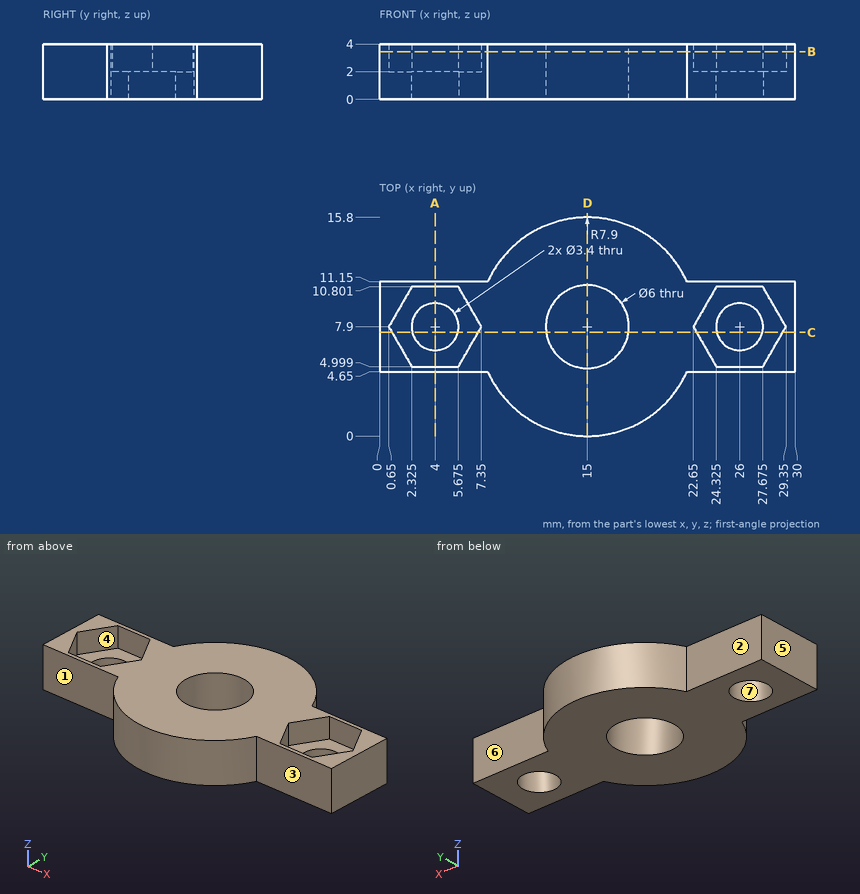
Drawing for the job (mm, zero at the part's lowest x, y, z). A direction names the side the tool comes from. Round coordinates to 2 decimals unless told otherwise and drop trailing zeros. Order: outer loops, then holes, each group sorted by start corner. A loop starts at its lowest first (then second) coordinate and runs counter-clockwise, first axis right, second up. Notation, with made-up numbers: (-28.75, 61) -> (23.25, 61) arc R19 ccw to (23.25, 69) -> close; hole circle Ø7 at (2.5, -24). An arc over 180 degrees is marked (long way). Write item = value, one per line. Start each with the question number.
(1) Cut at C-C, the plane y = 7.5. List the corners of the cut face in (x, z).
(2) Cut at A-A, the plane x = 4. List the corners of the cut face in (y, z).
(3) Cut at B-B, the plane z = 3.45. State how many separate pieces and enclosed holes the cut face has, then the cut area to 3 significant figures.
(4) Cut at D-D, the plane x = 15. List the corners of the cut face in (y, z).
(5) Which spindle directions (+Z, -Z, +X, -X, +Y, -Y) get a long thin tool onto all of the face, cutting with end or side? Do the marked faces 1, 2, 3 and 4. Say none if no direction does.
(6) Pull direction Y, two halves, no side cores. Call the marked faces 5, 6 and 7: released by +Y, released by -Y, zero draft, split by the parting line, or undercut.
(7) Probe line 1 (Y direction, x = 26, z = 1.1); line 2 (X direction, y = 7, z = 3.5); line 3 (Y direction, x = 15, z = 3.1). List the from-to ranges inside material, lowest first. Write a range as [from, to].
(8) Pin check, flat tips, straight feed: P1, Ø0.6, axis at x = 4.5, z = 3.5, coming from the +Y side; P2, Ø2, axis at x = 12.5, z = 1.5, coming from the -Y side; P3, Ø5.5, axis at x = 26, y = 7.9, coming from the +Z side; P4, Ø4.5, axis at x = 2.5, y = 7.5, coming from the +Z side. Stop position of each tip, or through.
Model answer:
q1.outline = (0, 0) -> (2.35, 0) -> (2.35, 2) -> (0.88, 2) -> (0.88, 4) -> (0, 4) -> close; (5.65, 0) -> (12.03, 0) -> (12.03, 4) -> (7.12, 4) -> (7.12, 2) -> (5.65, 2) -> close; (17.97, 0) -> (24.35, 0) -> (24.35, 2) -> (22.88, 2) -> (22.88, 4) -> (17.97, 4) -> close; (27.65, 0) -> (30, 0) -> (30, 4) -> (29.12, 4) -> (29.12, 2) -> (27.65, 2) -> close
q2.outline = (4.65, 0) -> (6.2, 0) -> (6.2, 2) -> (5, 2) -> (5, 4) -> (4.65, 4) -> close; (9.6, 0) -> (11.15, 0) -> (11.15, 4) -> (10.8, 4) -> (10.8, 2) -> (9.6, 2) -> close
q3.separate_pieces = 1
q3.enclosed_holes = 3
q3.area = 205 mm2
q4.outline = (0, 0) -> (4.9, 0) -> (4.9, 4) -> (0, 4) -> close; (10.9, 0) -> (15.8, 0) -> (15.8, 4) -> (10.9, 4) -> close
q5.face_1 = +Z, -Z, -X, -Y
q5.face_2 = +Z, -Z, -X, +Y
q5.face_3 = +Z, -Z, +X, -Y
q5.face_4 = +Z
q6.face_5 = zero draft
q6.face_6 = released by +Y
q6.face_7 = undercut
q7.line_1 = [4.65, 6.2], [9.6, 11.15]
q7.line_2 = [0, 1.17], [6.83, 12.14], [17.86, 23.17], [28.83, 30]
q7.line_3 = [0, 4.9], [10.9, 15.8]
q8.P1 = 11.15
q8.P2 = 0.14
q8.P3 = 2
q8.P4 = 4
